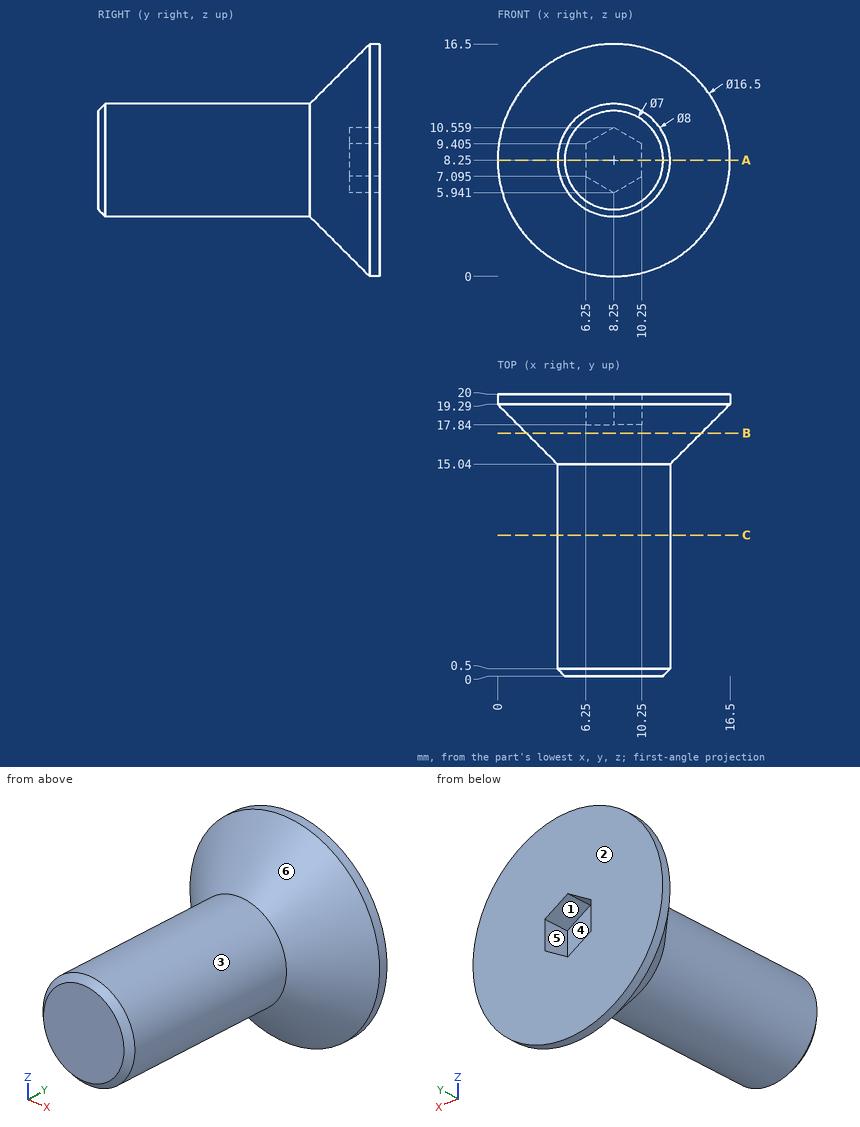
Design review of the part shown in the three views and the two pictorial views. Dimensions are in mm from the part's minimum x, y and z. A direction names the side the tool comes from. Coordinates: 2 decimals unless noted, no trailing zeros. Write each loop counter-clockwise with the first axis right and the second up, starting at its lowest first coordinate (ties: lowest second). Pieces come first, ordered by that corner, then holes.
(1) Wall thickness on probe 1 along Z at (x, y) = (9.75, 19) (1 decimal); probe 2 along Z at (x, y) = (7.5, 4.25); probe 3 along Z at (x, y) = (3, 18.5): over which ranges is each line inside the solid? List them lowest first.
(2) Tool access review of the marked faces 5 and 6: name each direction out of +Z, -Z, +X, -X, +Y, -Y from which nothing blocks a thin tool from reaching the whole face with its end or side.
(3) Add section A-A on z = 8.25. Give the boundary of the cut face in (x, y), then the cut area to 3 significant figures.
(4) Add section C-C on y = 10. Give the boundary of the cut face in (x, z).
(5) The part is to be moulded in two halves that separate along X. For the marked faces 1, 2, 3 and 4, say which applies: +X half, -X half, draft (parallel to the pull), parting line (faces both ways), or undercut.
(6) Add section B-B on y = 17.25. Give the boundary of the cut face in (x, z), then the cut area to 3 significant figures.
(7) For pin 1 Ø6 at (y, z) = (13, 8.5) entering from +X (1 decimal); pin 2 Ø6 at (x, y) = (11, 3.5) entering from +Z; pin 3 Ø8 at (x, y) = (10, 13) entering from +Z (1 decimal), all flat-tipped, find the tip position at first contact; note any pin that passes through.
Answer sheet:
1. probe 1: z = 0.4 to 6.8, 9.7 to 16.1
1. probe 2: z = 4.32 to 12.18
1. probe 3: z = 2.95 to 13.55
2. face 5: +Y
2. face 6: -Y
3. outline: (0, 19.29) - (4.25, 15.04) - (4.25, 0.5) - (4.75, 0) - (11.75, 0) - (12.25, 0.5) - (12.25, 15.04) - (16.5, 19.29) - (16.5, 20) - (10.25, 20) - (10.25, 17.84) - (6.25, 17.84) - (6.25, 20) - (0, 20) - close
3. area: 175 mm2
4. outline: circle Ø8 at (8.25, 8.25)
5. face 1: undercut
5. face 2: draft
5. face 3: parting line
5. face 4: undercut
6. outline: circle Ø12.42 at (8.25, 8.25)
6. area: 121 mm2
7. pin 1: stops at x = 13.2
7. pin 2: stops at z = 12.25
7. pin 3: stops at z = 14.1
